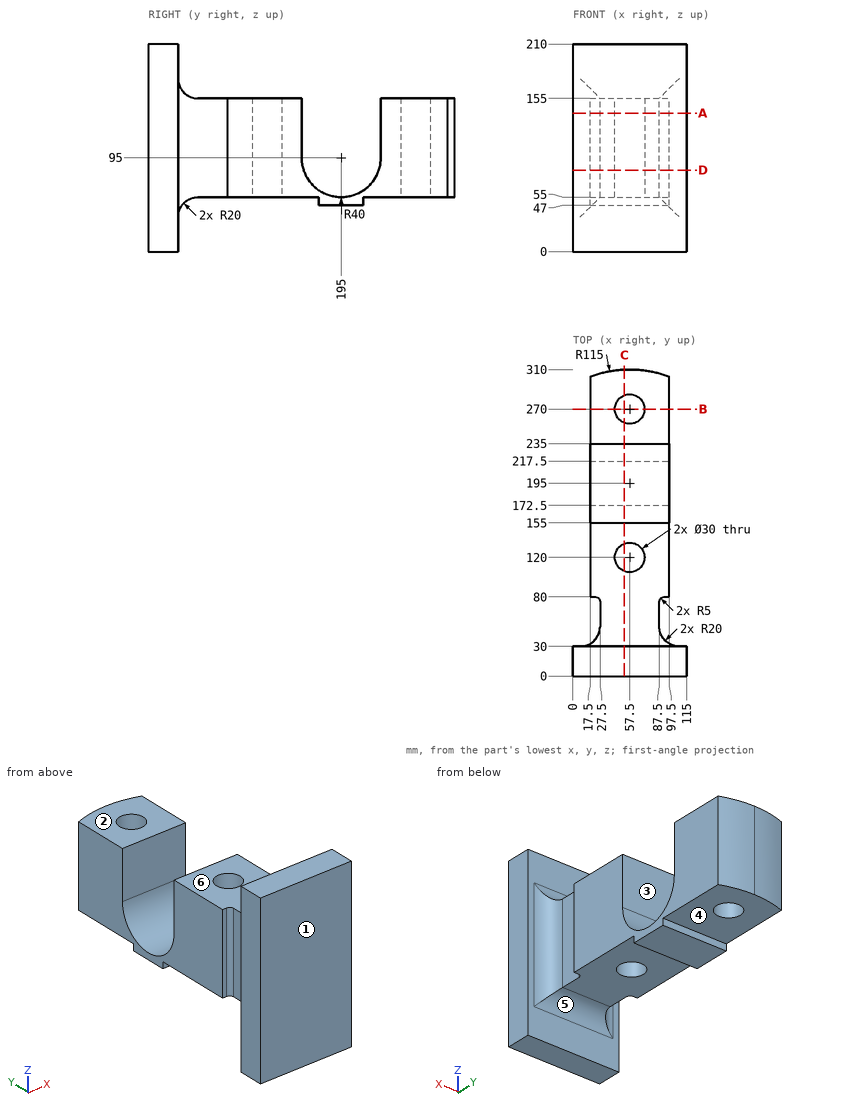
Geometry: see drawing. Coordinates: mm, zero at the bounding-box minimum. A direction names the side the tool comes from. Coordinates: 2 decimals unless noted, no trailing zeros. Write each loop counter-clockwise with the first axis right and the second up, starting at its lowest first coordinate (ties: lowest second). Pieces come first, ordered by that corner, then holes.
1) Material intervals for line 1 along Y through (x, z) = (57, 118); line 2 along Y through (x, z) = (19.5, 115); line 3 along Y through (x, z) = (48, 147.5), sorted ascending.
2) Mould query, pull axis Y, two halves, no side actions, for the marked faces 1, 2 and 3. Classes: pulls with the +Y half, pulls with the -Y half, needs draft (parallel to the pull), parting line crosses it, or undercut.
3) Section A-A on z = 140. Output: boundary loops of the cut face in (x, y), and give its area (3 significant figures).
4) Section B-B on y = 270. Output: boundary loops of the cut face in (x, z).
5) Section C-C on x = 52. Output: boundary loops of the cut face in (y, z), and give its area (3 significant figures).
6) Section D-D on z = 82.5. Output: boundary loops of the cut face in (x, y).
7) Set-up query: the marked faces 4, 5 and 6. Return all of +Z, -Z, +X, -X, +Y, -Y with unobstructed straight access to the full face (end or side cutting, diameter ignored); none if empty.
8) Pin query (flat end, axial travel): pin 1 Ø7.5 at (y, z) = (59, 106) entering from -X; pin 2 Ø1 at (y, z) = (245.5, 72) entering from +X; pin 3 Ø4 at (y, z) = (44.5, 58) entering from -X. Return the tip coordinate at first contact, or that it passes through.
Check result:
1. line 1: y = 0 to 105.01, 134.99 to 155, 235 to 255.01, 284.99 to 310
1. line 2: y = 0 to 34, 80 to 155, 235 to 303.54
1. line 3: y = 0 to 108.39, 131.61 to 155, 235 to 258.39, 281.61 to 309.61
2. face 1: pulls with the -Y half
2. face 2: needs draft
2. face 3: undercut
3. outline: (0, 0) - (115, 0) - (115, 30) - (107.5, 30) arc R20 cw to (87.5, 50) - (87.5, 75) arc R5 cw to (92.5, 80) - (97.5, 80) - (97.5, 155) - (17.5, 155) - (17.5, 80) - (22.5, 80) arc R5 cw to (27.5, 75) - (27.5, 50) arc R20 cw to (7.5, 30) - (0, 30) - close; (17.5, 235) - (97.5, 235) - (97.5, 302.82) arc R115 ccw to (17.5, 302.82) - close; hole circle Ø30 at (57.5, 120); hole circle Ø30 at (57.5, 270)
3. area: 17,000 mm2
4. outline: (17.5, 55) - (42.5, 55) - (42.5, 155) - (17.5, 155) - close; (72.5, 55) - (97.5, 55) - (97.5, 155) - (72.5, 155) - close
5. outline: (0, 0) - (30, 0) - (30, 35) arc R20 cw to (50, 55) - (106.04, 55) - (106.04, 155) - (50, 155) arc R20 cw to (30, 175) - (30, 210) - (0, 210) - close; (133.96, 55) - (172.5, 55) - (172.5, 47) - (217.5, 47) - (217.5, 55) - (256.04, 55) - (256.04, 155) - (235, 155) - (235, 95) arc R40 cw to (155, 95) - (155, 155) - (133.96, 155) - close; (283.96, 55) - (309.87, 55) - (309.87, 155) - (283.96, 155) - close
5. area: 21,900 mm2
6. outline: (0, 0) - (115, 0) - (115, 30) - (107.5, 30) arc R20 cw to (87.5, 50) - (87.5, 75) arc R5 cw to (92.5, 80) - (97.5, 80) - (97.5, 157) - (17.5, 157) - (17.5, 80) - (22.5, 80) arc R5 cw to (27.5, 75) - (27.5, 50) arc R20 cw to (7.5, 30) - (0, 30) - close; (17.5, 233) - (97.5, 233) - (97.5, 302.82) arc R115 ccw to (17.5, 302.82) - close; hole circle Ø30 at (57.5, 120); hole circle Ø30 at (57.5, 270)
7. face 4: -Z, +X, -X, +Y
7. face 5: -Z, +X, -X
7. face 6: +Z, +X, -X, +Y
8. pin 1: stops at x = 27.5
8. pin 2: stops at x = 97.5
8. pin 3: stops at x = 26.04
